Input: part model. Units: mm. Frame: model coordinates. A direction names the side the tool comes from. Round coordinates to 2 decimals unless told otherwise and drop trailing zeros. Write each loop counter-clockwise with the first axis right and the second up, starting at its lowest first coordinate (ties: lowest second). Pieces come first, ordered by that corner, then holes. Notation, with made-up numbers: (35.25, 15) -> (39.25, 15) arc R27 ccw to (39.25, 44) -> close; hole circle Ø5 at (11, 59). An arc over 180 degrees is marked (long way). Use CSV: the item, a comma, the result in double quotes.
```python
from build123d import *

# Parameters (mm, degrees)
F0_R     = 14.65
F1_DEPTH = 14
F2_R     = 2.4
F2_R_2   = 0.7
F3_DEPTH = 2.8
F4_R     = 3.5
F4_R_2   = 2.5
F5_DEPTH = 25
F7_DEPTH = 2


# Not quite as in the source:
# - a feature of the source that left no trace in its solid (it failed there, or was rolled back) is left out


with BuildPart() as f1:
    # F0 (on Top) → F1 (new body)
    with BuildSketch(Plane.XY):
        Circle(F0_R)
    extrude(amount=F1_DEPTH)

    # F2 (on face) → F3 (join)
    with BuildSketch(Plane(origin=(0, 0, 0), x_dir=(1, 0, 0), z_dir=(0, 0, -1))):
        with Locations((0, 12)):
            Circle(F2_R)
        with Locations((0, 12)):
            Circle(F2_R_2, mode=Mode.SUBTRACT)
        with Locations((-10.3923048454, -6)):
            Circle(F2_R)
        with Locations((-10.3923048454, -6)):
            Circle(F2_R_2, mode=Mode.SUBTRACT)
        with Locations((10.3923048454, -6)):
            Circle(F2_R)
        with Locations((10.3923048454, -6)):
            Circle(F2_R_2, mode=Mode.SUBTRACT)
    extrude(amount=F3_DEPTH)

    # F4 (on face) → F5 (cut)
    with BuildSketch(Plane.XY.offset(14)):
        Circle(F4_R)
        with Locations((7.3377376988, -4.5508025283)):
            Circle(F4_R_2)
    extrude(amount=-F5_DEPTH, mode=Mode.SUBTRACT)

    # F6 (on face) → F7 (cut)
    with BuildSketch(Plane.XY.offset(14)):
        with BuildLine():
            ThreePointArc((3.265158964, -1.5745989775), (3.533894894, -0.8075963582), (3.625, 0))
            ThreePointArc((3.625, 0), (3.533894894, 0.8075963582), (3.265158964, 1.5745989775))
            ThreePointArc((3.265158964, 1.5745989775), (0, 3.625), (-3.265158964, 1.5745989775))
            ThreePointArc((-3.265158964, 1.5745989775), (-3.625, 0), (-3.265158964, -1.5745989775))
            ThreePointArc((-3.265158964, -1.5745989775), (0, -3.625), (3.265158964, -1.5745989775))
        make_face()
        with BuildLine():
            ThreePointArc((-3.265158964, 1.5745989775), (0, 3.625), (3.265158964, 1.5745989775))
            Line((3.265158964, 1.5745989775), (2.0405680426, 14.2964231749))
            ThreePointArc((2.0405680426, 14.2964231749), (2.047640653, 14.1983247495), (2.05, 14.1))
            ThreePointArc((2.05, 14.1), (-0.0983247495, 12.052359347), (-2.0405680426, 14.2964231749))
            Line((-2.0405680426, 14.2964231749), (-3.265158964, 1.5745989775))
        make_face()
        with BuildLine():
            Line((2.0405680426, -14.2964231749), (3.265158964, -1.5745989775))
            ThreePointArc((3.265158964, -1.5745989775), (0, -3.625), (-3.265158964, -1.5745989775))
            Line((-3.265158964, -1.5745989775), (-2.0405680426, -14.2964231749))
            ThreePointArc((-2.0405680426, -14.2964231749), (-0.0983247495, -12.052359347), (2.05, -14.1))
            ThreePointArc((2.05, -14.1), (2.047640653, -14.1983247495), (2.0405680426, -14.2964231749))
        make_face()
        with BuildLine():
            ThreePointArc((2.05, 14.1), (2.047640653, 14.1983247495), (2.0405680426, 14.2964231749))
            ThreePointArc((2.0405680426, 14.2964231749), (0, 16.15), (-2.0405680426, 14.2964231749))
            ThreePointArc((-2.0405680426, 14.2964231749), (-0.0983247495, 12.052359347), (2.05, 14.1))
        make_face()
        with BuildLine():
            ThreePointArc((-2.0405680426, -14.2964231749), (0, -16.15), (2.0405680426, -14.2964231749))
            ThreePointArc((2.0405680426, -14.2964231749), (2.047640653, -14.1983247495), (2.05, -14.1))
            ThreePointArc((2.05, -14.1), (-0.0983247495, -12.052359347), (-2.0405680426, -14.2964231749))
        make_face()
    extrude(amount=-F7_DEPTH, mode=Mode.SUBTRACT)


solid = f1.part
```
Item 1: Pull-direction query (X, two-part tool) for faces 1 (the face through (11, 5, -2.8)), 2 (the face through (1.29, -14.024, -1.38)), 3 (the face through (0, -12, 0)); classes: +X half, -X half, draft (parallel to the pull), parting line (faces both ways), or undercut.
Worked answers:
face 1,"draft"
face 2,"parting line"
face 3,"undercut"
Item 2: Section query D-D on x = 7. Return the cut outline in (y, z).
Worked answers:
outline,"(-12.87, 0) -> (-7.03, 0) -> (-7.03, 14) -> (-12.87, 14) -> close; (-2.07, 0) -> (12.87, 0) -> (12.87, 14) -> (-2.07, 14) -> close"
Item 3: Section query A-A on x = 0. Return the cut outline in (y, z), plus the area to 3 significant figures.
Worked answers:
outline,"(-14.65, 0) -> (-14.4, 0) -> (-14.4, -2.8) -> (-12.7, -2.8) -> (-12.7, 0) -> (-11.3, 0) -> (-11.3, -2.8) -> (-9.6, -2.8) -> (-9.6, 0) -> (-3.5, 0) -> (-3.5, 12) -> (-14.65, 12) -> close; (3.5, 0) -> (14.65, 0) -> (14.65, 12) -> (3.5, 12) -> close"
area,"277 mm²"
Item 4: Line query: line 1 (Y direction, x = 0, z = -1.35); line 2 (Y direction, x = 0, z = 6.75); line 3 (X direction, y = -12, z = -0.8). Output: solid intervals per line, ascending.
Worked answers:
line 1,"y = -14.4 to -12.7, -11.3 to -9.6"
line 2,"y = -14.65 to -3.5, 3.5 to 14.65"
line 3,"x = -2.4 to -0.7, 0.7 to 2.4"
Item 5: Section query C-C on y = 12.5. Return the cut outline in (x, z), plus the area to 3 significant figures.
Worked answers:
outline,"(-7.64, 0) -> (7.64, 0) -> (7.64, 14) -> (2.21, 14) -> (2.21, 12) -> (-2.21, 12) -> (-2.21, 14) -> (-7.64, 14) -> close"
area,"205 mm²"
Item 6: Set-up query: faces 4 (the face through (-9.1, 3.98, -1.38)), 5 (the face through (-1, -12, -2.8)), 6 (the face through (-3.625, 0.023, 13.014)). Return all of +Z, -Z, +X, -X, +Y, -Y with unobstructed straight access to the full face (end or side cutting, diameter ignored); none if empty.
Worked answers:
face 4,"-Z"
face 5,"-Z, +X, -X, +Y, -Y"
face 6,"+Z"
Item 7: First-contact query: pin 1 Ø2 at (y, z) = (5, 4.5) entering from +X; pin 2 Ø10 at (x, z) = (8.5, 1) entering from +Y; pin 3 Ø4 at (y, z) = (10.5, 10) entering from +X. Flat tips, straight axial feed; report the tip coordinate or a pass-through.
Worked answers:
pin 1,"stops at x = 14.09"
pin 2,"stops at y = 14.23"
pin 3,"stops at x = 11.93"
Item 8: Section query B-B on y = -5.75. Return the cut outline in (x, z), plus the area to 3 significant figures.
Worked answers:
outline,"(-13.47, 0) -> (5.14, 0) -> (5.14, 14) -> (2.86, 14) -> (2.86, 12) -> (-2.86, 12) -> (-2.86, 14) -> (-13.47, 14) -> close; (9.53, 0) -> (13.47, 0) -> (13.47, 14) -> (9.53, 14) -> close"
area,"304 mm²"
